Geometry: see drawing. Coordinates: mm, zero at the bounding-box minimum. A direction names the side the tool comes from. Give positions to 0.01 mm unless a question says otherwise; leave off trailing zeros. Loops run counter-clockwise (first coordinate to the right, second up) from the corner with the lowest first, then second, coordinate; pieces in that order, holes last. Notation, with made-up numbers: (32, -19) - (73, -19) arc R34 ccw to (73, 11) - close; hole circle Ø6 at (17, 75.5). An arc over 180 degrees is marked (long way). Use CSV: the item, a comma, the result in double quotes. Start each with the question number.
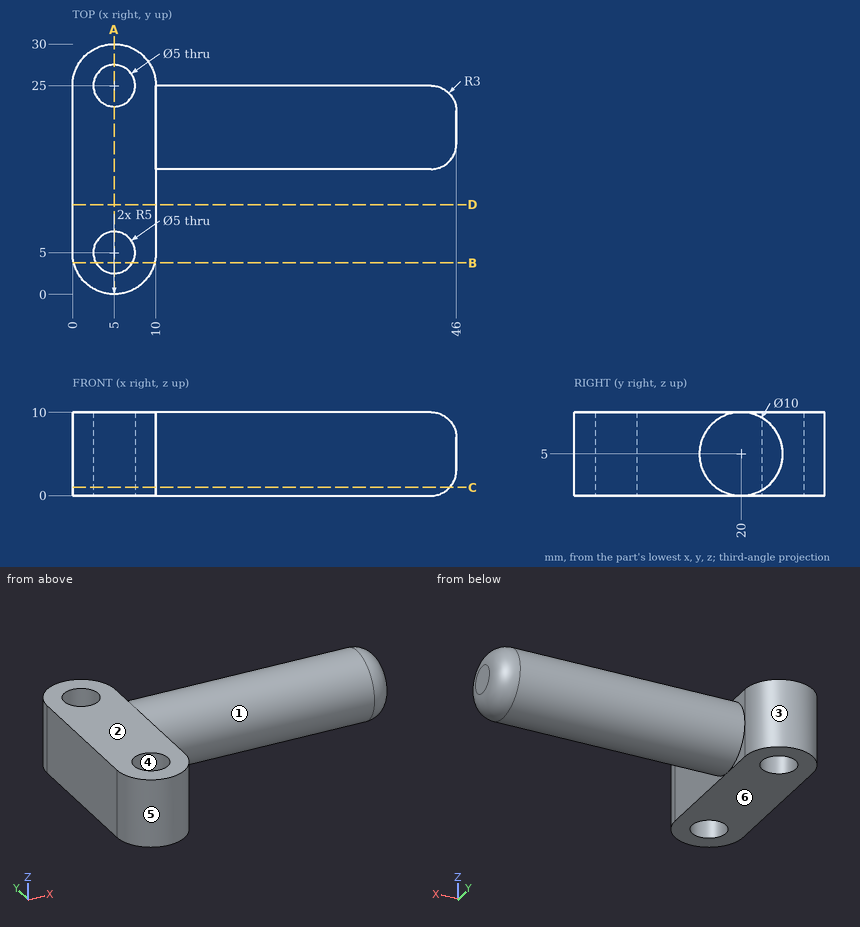
Item 1: Section C-C (z = 1). Give the number of separate pieces and of enclosed holes in the cut face, plus the area to 3 significant figures.
Item 2: Mould query, pull axis Y, two halves, no side actions, for the marked faces 3, 4, 5 and 6. Classes: pulls with the +Y half, pulls with the -Y half, needs draft (parallel to the pull), parting line crosses it, or undercut.
Item 3: Pin query (flat end, axial travel): pin 1 Ø3 at (x, z) = (10.5, 4.5) entering from -Y; pin 2 Ø8 at (x, y) = (17.5, 9.5) entering from -Z; pin 3 Ø1.5 at (y, z) = (13.5, 3) entering from +X; pin 4 Ø4 at (x, z) = (38, 1.5) entering from +Y. Return the tip coordinate at first contact, or that it passes through.
Item 4: Reachability of the marked faces 1 and 2 from +Z, -Z, +X, -X, +Y, -Y: full face, straight path, thin tool, end or side. Return the list, or none.
Item 5: Section A-A (x = 5). Output: boundary loops of the cut face in (y, z), plus the area to 3 significant figures.
Item 6: Section D-D (y = 10.75). Output: boundary loops of the cut face in (x, z), plus the area to 3 significant figures.
Item 7: Ray query, probe 1 along Y at (x, z) = (5, 6); probe 2 along X at (y, z) = (23.5, 1.25); probe 3 along X at (y, z) = (15, 6.25). Return the intervals inside material, ascending.
Item 8: Section B-B (y = 3.75). Output: boundary loops of the cut face in (x, z), plus the area to 3 significant figures.
Outcome:
1,separate pieces,"1"
1,enclosed holes,"2"
1,area,"448 mm2"
2,face 3,"pulls with the +Y half"
2,face 4,"undercut"
2,face 5,"pulls with the -Y half"
2,face 6,"needs draft"
3,pin 1,"stops at y = 2"
3,pin 2,"passes through"
3,pin 3,"stops at x = 10"
3,pin 4,"stops at y = 24.77"
4,face 1,"+X"
4,face 2,"+Z, +X, -X, +Y, -Y"
5,outline,"(0, 0) - (2.5, 0) - (2.5, 10) - (0, 10) - close; (7.5, 0) - (22.5, 0) - (22.5, 10) - (7.5, 10) - close; (27.5, 0) - (30, 0) - (30, 10) - (27.5, 10) - close"
5,area,"200 mm2"
6,outline,"(0, 0) - (10, 0) - (10, 10) - (0, 10) - close"
6,area,"100 mm2"
7,probe 1,"y = 0 to 2.5, 7.5 to 22.5, 27.5 to 30"
7,probe 2,"x = 0 to 3, 7 to 10"
7,probe 3,"x = 0 to 10"
8,outline,"(0.16, 0) - (2.83, 0) - (2.83, 10) - (0.16, 10) - close; (7.17, 0) - (9.84, 0) - (9.84, 10) - (7.17, 10) - close"
8,area,"53.5 mm2"
